Verification items for this drawing (mm, ordinates from the low corner). Give positions to 0.01 mm unless a question says otherwise; leave off trailing zeros. Order: outer loops, then holes, each group sorted by start corner. A loop starts at its lowest first (then second) coordinate and runs counter-clockwise, first axis right, second up.
(1) Sectioned sample at C-C on z = 265. Record the cut outline in (x, y), plus the area to 3 significant figures.
(2) Sectioned sample at B-B on x = 268. Record the cut outline in (y, z).
(3) Sectioned sample at A-A on y = 12. Record the cut outline in (x, z), plus the area to 3 significant figures.
(4) Scan lines: L1, parallel to Z at x = 574.5, y = 5.25; L2, parallel to X at y = 9.25, z = 38.5; L3, parallel to Z at x = 238.5, y = 6.5. Record each from-to range of solid material in increasing order.
(5) Gauge pin test, flat ends, axial feed: pin 1 (1.5 mm diameter, centred on x = 300, y = 15, fed in from -Z); pin 2 (10 mm diameter, centred on x = 167.5, y = 12.5, fed in from +Z); pin 3 (5 mm diameter, centred on y = 8, z = 80, fed in from -X). Record the tip position at first contact, or that the pin passes through.
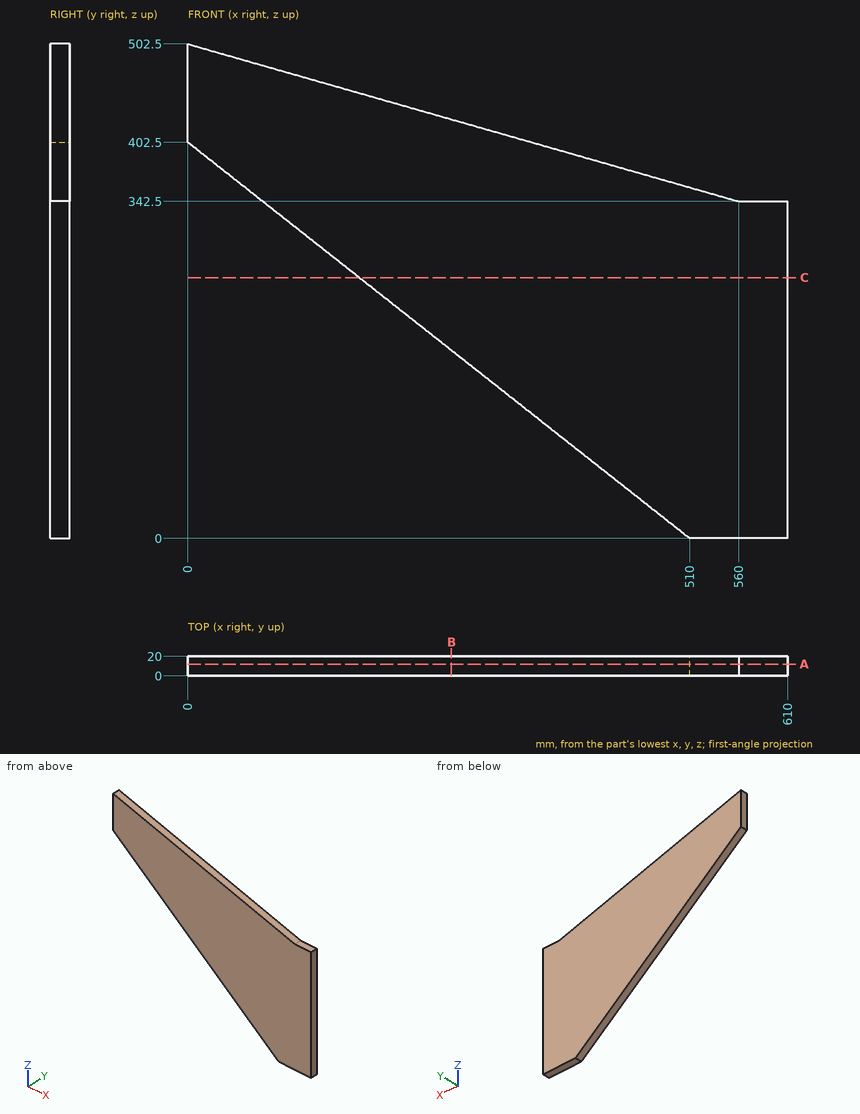
Ans:
1. outline: (174.22, 0) - (610, 0) - (610, 20) - (174.22, 20) - close
1. area: 8,720 mm2
2. outline: (0, 190.99) - (20, 190.99) - (20, 425.93) - (0, 425.93) - close
3. outline: (0, 402.5) - (510, 0) - (610, 0) - (610, 342.5) - (560, 342.5) - (0, 502.5) - close
3. area: 151,000 mm2
4. L1: z = 0 to 342.5
4. L2: x = 461.22 to 610
4. L3: z = 214.27 to 434.36
5. pin 1: stops at z = 165.14
5. pin 2: stops at z = 456.07
5. pin 3: stops at x = 405.47
